```python
from build123d import *

# Parameters (mm, degrees)
SKETCH_1_R               = 5.5
EXTRUDE_1_DEPTH          = 1.1
CUT_EXTRUDE_1_DEPTH      = 12.175419455
CUT_EXTRUDE_1_DEPTH_BACK = 1.1
SKETCH_2_W               = 2
SKETCH_2_H               = 8.74586507
SKETCH_3_R               = 0.75
CUT_EXTRUDE_1_2_DEPTH    = 12.130588484


with BuildPart() as part:
    # 草图1 → 凸台-拉伸1 (new body)
    with BuildSketch(Plane.XY):
        with BuildLine():
            Line((-5, -4.339608214), (-4.423832973, -7.607213802))
            ThreePointArc((-4.423832973, -7.607213802), (0, -8.8), (4.423832973, -7.607213802))
            Line((4.423832973, -7.607213802), (5, -4.339608214))
            ThreePointArc((5, -4.339608214), (6.257657716, -2.319610394), (6.788225099, 0))
            ThreePointArc((6.788225099, 0), (0, 7.2), (-6.788225099, 0))
            ThreePointArc((-6.788225099, 0), (-6.257657716, -2.319610394), (-5, -4.339608214))
        make_face()
        Circle(SKETCH_1_R, mode=Mode.SUBTRACT)
    extrude(amount=EXTRUDE_1_DEPTH)

    # 草图2 → Cut-Extrude 1 (cut, two sides: drawn at the far end of the back side and taken through both)
    with BuildSketch(Plane.XY.offset(1.1).offset(-CUT_EXTRUDE_1_DEPTH_BACK)):
        with Locations((0, -8.997615825)):
            Rectangle(SKETCH_2_W, SKETCH_2_H)
    extrude(amount=CUT_EXTRUDE_1_DEPTH + CUT_EXTRUDE_1_DEPTH_BACK, mode=Mode.SUBTRACT)

    # 草图3 → Cut-Extrude 1 2 (cut, through all)
    with BuildSketch(Plane.XY.offset(1.1)):
        with Locations((3, -6.801492871)):
            Circle(SKETCH_3_R)
        with Locations((-3, -6.801492871)):
            Circle(SKETCH_3_R)
    extrude(amount=-CUT_EXTRUDE_1_2_DEPTH, mode=Mode.SUBTRACT)


solid = part.part
```
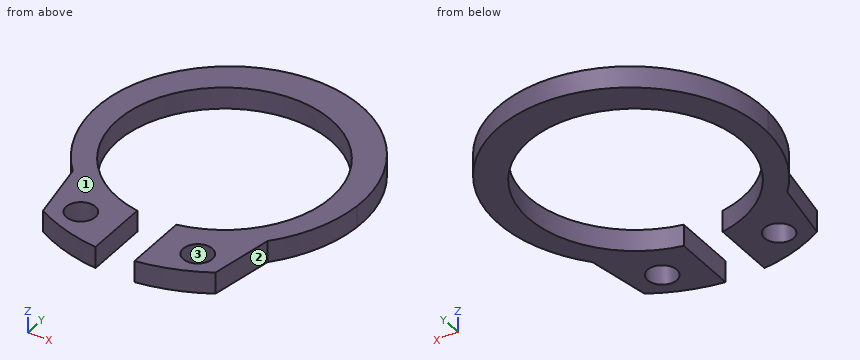
Source: CAD feature listing. Evaluate the final solid. Frame: model axes, mm. Face numbers are marked on the shaded views. Give positions to 0.01 mm unless a question says otherwise; leave off trailing zeros. Loops run counter-clockwise (first coordinate to the right, second up) from the corner with the lowest first, then second, coordinate; pieces in that order, holes last. Notation, with made-up numbers: (83.5, 24.5) -> (128.5, 24.5) arc R31 ccw to (128.5, 52.5) -> close; hole circle Ø3 at (66, 31.5). An arc over 180 degrees is marked (long way). Use a Markdown table: item, result. Add a question column.
(1) Section query D-D (x = 3). Output: boundary loops of the cut face in (y, z).
(2) Section query C-C (z = 0.85). Output: boundary loops of the cut face in (x, y).
(3) Section query A-A (y = 0.4). Output: boundary loops of the cut face in (x, z).
(4) Pull-direction query (X, two-part tool) for the marked faces 1, 2 and 3; classes: +X half, -X half, draft (parallel to the pull), parting line (faces both ways), or undercut.
(5) Ray query, line 1 (Y direction, x = -3, z = 0.8); line 2 (Y direction, x = 2.75, z = 0.4); line 3 (X direction, y = -7, z = 0.55). Return the intervals inside material, ascending.
(6) First-contact query: pin 1 Ø2.5 at (x, y) = (-3, -6.8) entering from +Z. Flat tip, straight axial feed; report the tip coordinate or a pass-through.
(7) Section query B-B (x = -4.25). Output: boundary loops of the cut face in (y, z), then the cut area to 4 significant figures.
Checked values:
| question | item | result |
|---|---|---|
| 1 | outline | (-8.27, 0) -> (-7.55, 0) -> (-7.55, 1.1) -> (-8.27, 1.1) -> close; (-6.05, 0) -> (-4.61, 0) -> (-4.61, 1.1) -> (-6.05, 1.1) -> close; (4.61, 0) -> (6.5, 0) -> (6.5, 1.1) -> (4.61, 1.1) -> close |
| 2 | outline | (-6.79, 0) arc R7.2 ccw to (-5, -4.34) -> (-4.42, -7.61) arc R8.8 ccw to (-1, -8.74) -> (-1, -5.41) arc R5.5 cw (long way) to (1, -5.41) -> (1, -8.74) arc R8.8 ccw to (4.42, -7.61) -> (5, -4.34) arc R7.2 ccw to (6.79, 0) arc R6.8 ccw (long way) to start; hole circle Ø1.5 at (-3, -6.8); hole circle Ø1.5 at (3, -6.8) |
| 3 | outline | (-6.8, 0) -> (-5.49, 0) -> (-5.49, 1.1) -> (-6.8, 1.1) -> close; (5.49, 0) -> (6.8, 0) -> (6.8, 1.1) -> (5.49, 1.1) -> close |
| 4 | face 1 | draft |
| 4 | face 2 | +X half |
| 4 | face 3 | undercut |
| 5 | line 1 | -8.27 to -7.55, -6.05 to -4.61, 4.61 to 6.5 |
| 5 | line 2 | -8.36 to -7.51, -6.09 to -4.76, 4.76 to 6.62 |
| 5 | line 3 | -4.53 to -3.72, -2.28 to -1, 1 to 2.28, 3.72 to 4.53 |
| 6 | pin 1 | z = 1.1 |
| 7 | outline | (-7.71, 0) -> (-3.49, 0) -> (-3.49, 1.1) -> (-7.71, 1.1) -> close; (3.49, 0) -> (5.71, 0) -> (5.71, 1.1) -> (3.49, 1.1) -> close |
| 7 | area | 7.075 mm^2 |
